Could you check a few things on this model? Use its own coordinates, in mm. Coordinates: 2 decimals unless noted, no trailing zeros. Order: outer loops, then holes, each group sorted by start corner. A loop starts at its lowest first (then second) coordinate and runs counter-clockwise, first axis right, second up. Notation, with made-up numbers: (-9.75, 51.5) - (-2.75, 51.5) arc R26 cw to (-2.75, 77.5) - close; hole circle Ø5 at (9, 68). An arc over 180 degrees is marked (long way). Answer as a JSON object with one key per item and string values. Group by question number.
(1) Imagine slicing it at B-B, the plane y = -3. Write out the boundary of the cut face in (x, z), and give its area (3 significant figures).
(2) Imagine slicing it at A-A, the plane z = 8.5. Write out the boundary of the cut face in (x, y) (3 decimals).
(3) Imagine slicing it at D-D, the plane x = 1.2. Give the number of separate pieces and of enclosed holes in the cut face, and give its area (3 significant figures).
(4) Please list where these lines run through material, in increasing order: probe 1 along Y at (x, z) = (0.25, 6) (3 decimals); probe 2 along Y at (x, z) = (1.8, 4) (3 decimals); probe 3 along Z at (x, y) = (0.55, 8.5).
(5) Will these pins go through, and if not, where does the flat tip stop? P1, Ø1, axis at x = 1, y = -5, coming from the -Z side; P2, Ø1, axis at x = 1, y = -4.5, coming from the +Z side; P3, Ø0.6, axis at x = 1.5, z = -40, coming from the -Y side.
(6) Imagine slicing it at C-C, the plane y = 10.25. Write out the boundary of the cut face in (x, z), and give its area (3 significant figures).
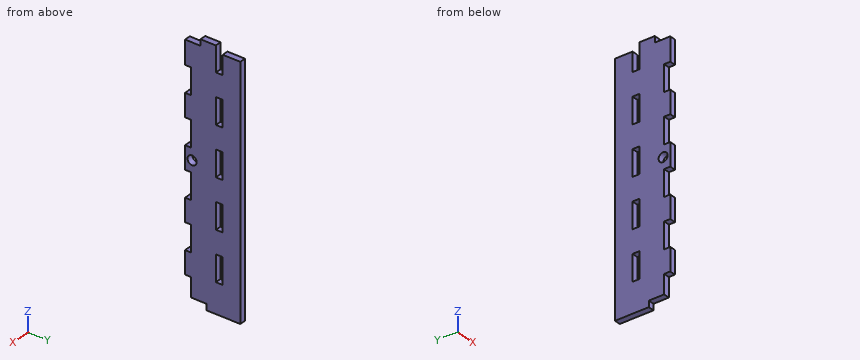
from build123d import *

# Parameters (mm, degrees)
ESQUISSE1_W             = 82
ESQUISSE1_H             = 12.11
BOSS_EXTRU_1_DEPTH      = 2
ESQUISSE2_W             = 8.5
ESQUISSE2_H             = 2.25
ENL_V_MAT_EXTRU_1_DEPTH = 42.581069992
ESQUISSE3_W             = 8.5
ESQUISSE3_H             = 2
ENL_V_MAT_EXTRU_2_DEPTH = 42.581069992
ESQUISSE4_W             = 2
ESQUISSE4_H             = 5.055
ENL_V_MAT_EXTRU_3_DEPTH = 42.581069992
ESQUISSE5_W             = 80
ESQUISSE5_H             = 6
BOSS_EXTRU_2_DEPTH      = 2
ESQUISSE6_W             = 6.25
ESQUISSE6_H             = 0.25
ESQUISSE6_W_2           = 8.5
ENL_V_MAT_EXTRU_4_DEPTH = 43.867766231
SKETCH1_R               = 1.5
CUT_EXTRUDE1_DEPTH      = 43.867766231


with BuildPart() as part:
    # Esquisse1 → Boss.-Extru.1 (new body)
    with BuildSketch(Plane(origin=(0, 0, 0), x_dir=(0, 0, -1), z_dir=(1, 0, 0))):
        with Locations((-0.0892, 0)):
            Rectangle(ESQUISSE1_W, ESQUISSE1_H)
    extrude(amount=BOSS_EXTRU_1_DEPTH)

    # Esquisse2 → Enlèv. mat.-Extru.1 (cut, through all)
    with BuildSketch(Plane(origin=(0, 0, 0), x_dir=(0, 0, -1), z_dir=(1, 0, 0))):
        with Locations((-37.0892, 5.18)):
            Rectangle(ESQUISSE2_W, ESQUISSE2_H)
        with Locations((-21.0892, 5.18)):
            Rectangle(ESQUISSE2_W, ESQUISSE2_H)
        with Locations((-5.0892, 5.18)):
            Rectangle(ESQUISSE2_W, ESQUISSE2_H)
        with Locations((10.9108, 5.18)):
            Rectangle(ESQUISSE2_W, ESQUISSE2_H)
        with Locations((26.9108, 5.18)):
            Rectangle(ESQUISSE2_W, ESQUISSE2_H)
    extrude(amount=ENL_V_MAT_EXTRU_1_DEPTH, mode=Mode.SUBTRACT)

    # Esquisse3 → Enlèv. mat.-Extru.2 (cut, through all)
    with BuildSketch(Plane(origin=(0, 0, 0), x_dir=(0, 0, -1), z_dir=(1, 0, 0))):
        with Locations((-27.0892, -5.055)):
            Rectangle(ESQUISSE3_W, ESQUISSE3_H)
        with Locations((-11.0892, -5.055)):
            Rectangle(ESQUISSE3_W, ESQUISSE3_H)
        with Locations((4.9108, -5.055)):
            Rectangle(ESQUISSE3_W, ESQUISSE3_H)
        with Locations((20.9108, -5.055)):
            Rectangle(ESQUISSE3_W, ESQUISSE3_H)
        with Locations((36.9108, -5.055)):
            Rectangle(ESQUISSE3_W, ESQUISSE3_H)
    extrude(amount=ENL_V_MAT_EXTRU_2_DEPTH, mode=Mode.SUBTRACT)

    # Esquisse4 → Enlèv. mat.-Extru.3 (cut, through all)
    with BuildSketch(Plane(origin=(2, 0, 0), x_dir=(0, 0, -1), z_dir=(1, 0, 0))):
        with Locations((-40.0892, -3.5275)):
            Rectangle(ESQUISSE4_W, ESQUISSE4_H)
        with Locations((39.9108, -1.5275)):
            Rectangle(ESQUISSE4_W, ESQUISSE4_H)
    extrude(amount=-ENL_V_MAT_EXTRU_3_DEPTH, mode=Mode.SUBTRACT)

    # Esquisse5 → Boss.-Extru.2 (add)
    with BuildSketch(Plane.ZY):
        with Locations((-0.9108, 9.055)):
            Rectangle(ESQUISSE5_W, ESQUISSE5_H)
    extrude(amount=-BOSS_EXTRU_2_DEPTH)

    # Esquisse6 → Enlèv. mat.-Extru.4 (cut, through all)
    with BuildSketch(Plane(origin=(2, 0, 0), x_dir=(0, 0, -1), z_dir=(1, 0, 0))):
        with Locations((-35.9642, 6.18)):
            Rectangle(ESQUISSE6_W, ESQUISSE6_H)
        with Locations((-21.0892, 6.18)):
            Rectangle(ESQUISSE6_W_2, ESQUISSE6_H)
        with Locations((-5.0892, 6.18)):
            Rectangle(ESQUISSE6_W_2, ESQUISSE6_H)
        with Locations((10.9108, 6.18)):
            Rectangle(ESQUISSE6_W_2, ESQUISSE6_H)
        with Locations((26.9108, 6.18)):
            Rectangle(ESQUISSE6_W_2, ESQUISSE6_H)
    extrude(amount=-ENL_V_MAT_EXTRU_4_DEPTH, mode=Mode.SUBTRACT)

    # Sketch1 → Cut-Extrude1 (cut, through all)
    with BuildSketch(Plane(origin=(2, 0, 0), x_dir=(0, 0, -1), z_dir=(1, 0, 0))):
        with Locations((-3.0892, -3.725)):
            Circle(SKETCH1_R)
    extrude(amount=-CUT_EXTRUDE1_DEPTH, mode=Mode.SUBTRACT)


solid = part.part
Result set:
{
 "1": {"outline": "(0, -38.91) - (2, -38.91) - (2, 1.78) - (0, 1.78) - close; (0, 4.4) - (2, 4.4) - (2, 39.09) - (0, 39.09) - close", "area": "151 mm^2"},
 "2": {"outline": "(0, -4.055) - (2, -4.055) - (2, 4.055) - (0, 4.055) - close; (0, 6.305) - (2, 6.305) - (2, 12.055) - (0, 12.055) - close"},
 "3": {"separate pieces": "1", "enclosed holes": "5", "area": "1,270 mm^2"},
 "4": {"probe 1": "y = -6.055 to 4.055, 6.305 to 12.055", "probe 2": "y = -6.055 to -4.917, -2.533 to 4.055, 6.305 to 12.055", "probe 3": "z = -40.91 to 39.09"},
 "5": {"P1": "stops at z = -32.66", "P2": "stops at z = 39.09", "P3": "stops at y = 1"},
 "6": {"outline": "(0, -40.91) - (2, -40.91) - (2, 39.09) - (0, 39.09) - close", "area": "160 mm^2"}
}
